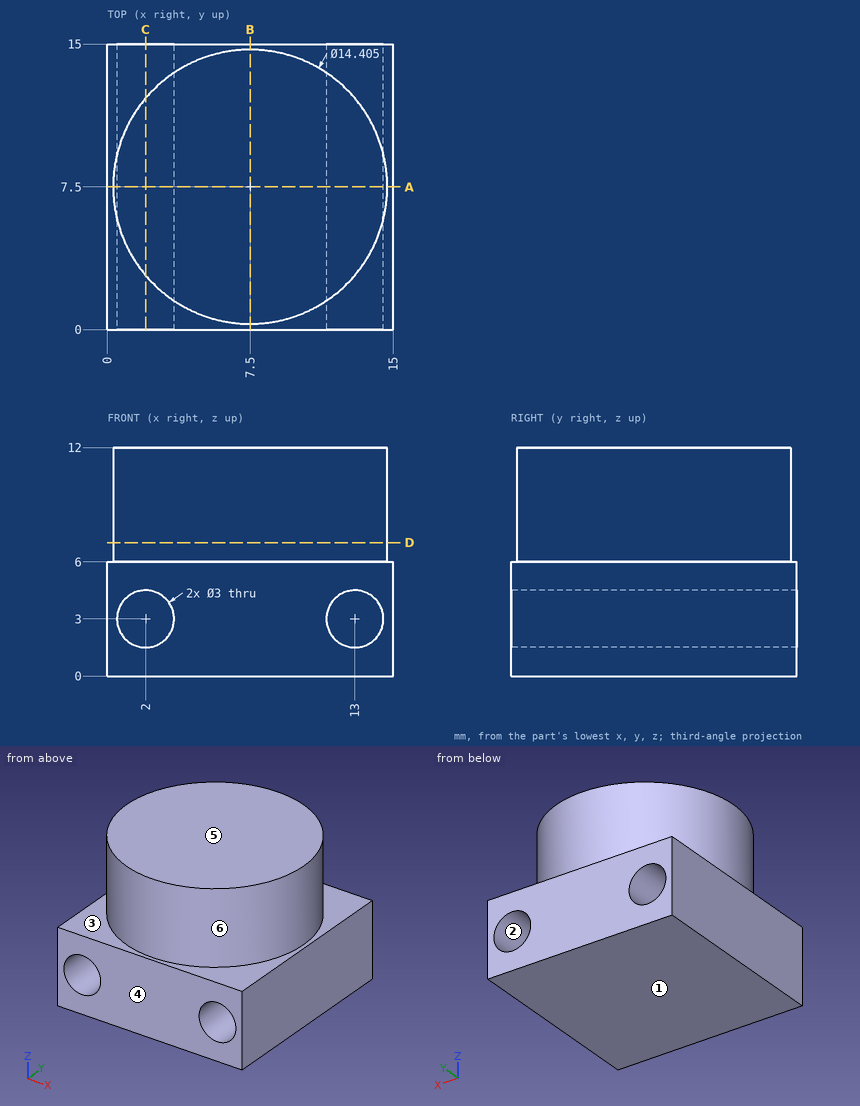
Check sheet for the drawn part. Datum: minimum x, y, z corner. Units: mm. A direction names the side the tool comes from. Coordinates: 2 decimals unless noted, no trailing zeros. Order: outer loops, then holes, each group sorted by start corner. A loop starts at its lowest first (then second) coordinate and runs counter-clockwise, first axis right, second up. Notation, with made-up numbers: M 26,66 L 64,66 A4 cw 64,71 Z; hole C -25.5,6.25 d6. An arc over 180 degrees is marked long. One line per item, written item: value. Start each with the question number.
Item 1: Sectioned sample at C-C (x = 2). Enter the section's corners in (y, z), then the cut area to 3 significant figures.
Item 2: Sectioned sample at D-D (z = 7). Enter the section's corners in (x, y) (1 decimal), then the cut area to 3 significant figures.
Item 3: Sectioned sample at B-B (x = 7.5). Enter the section's corners in (y, z).
Item 4: Access from +Z, -Z, +X, -X, +Y, -Y to the whole of each face (thin tool, end or side, straight path). Record for the marked faces 5 and 6.
Item 5: Gauge pin test, flat ends, axial feed: pin 1 (1.5 mm diameter, centred on y = 5.5, z = 8.5, fed in from -X); pin 2 (1.5 mm diameter, centred on y = 8, z = 7, fed in from +X). Record the tip position at first contact, or that the pin passes through.
Item 6: Scan lines: probe 1 along Z at (x, y) = (2, 9.5); probe 2 along X at (y, z) = (12.5, 3.25); probe 3 along Z at (x, y) = (12.5, 12.25). Record each from-to range of solid material in increasing order.
Item 7: Sectioned sample at A-A (y = 7.5). Enter the section's corners in (x, z), then the cut area to 3 significant figures.
Item 8: Mould release check, pull along Z, two halves, no side actions. Record for the marked faces 1, 2, 3 and 4: released by +Z, released by -Z, zero draft, split by the parting line, or undercut.
Conclusion:
1. outline: M 0,0 L 15,0 L 15,1.5 L 0,1.5 Z; M 0,4.5 L 15,4.5 L 15,6 L 12.15,6 L 12.15,12 L 2.85,12 L 2.85,6 L 0,6 Z
1. area: 101 mm^2
2. outline: C 7.5,7.5 d14.4
2. area: 163 mm^2
3. outline: M 0,0 L 15,0 L 15,6 L 14.7,6 L 14.7,12 L 0.3,12 L 0.3,6 L 0,6 Z
4. face 5: +Z, +X, -X, +Y, -Y
4. face 6: +Z
5. pin 1: stops at x = 0.41
5. pin 2: stops at x = 14.7
6. probe 1: z = 0 to 1.5, 4.5 to 12
6. probe 2: x = 0 to 0.52, 3.48 to 11.52, 14.48 to 15
6. probe 3: z = 0 to 1.59, 4.41 to 12
7. outline: M 0,0 L 15,0 L 15,6 L 14.7,6 L 14.7,12 L 0.3,12 L 0.3,6 L 0,6 Z; hole C 2,3 d3; hole C 13,3 d3
7. area: 162 mm^2
8. face 1: released by -Z
8. face 2: undercut
8. face 3: released by +Z
8. face 4: zero draft
